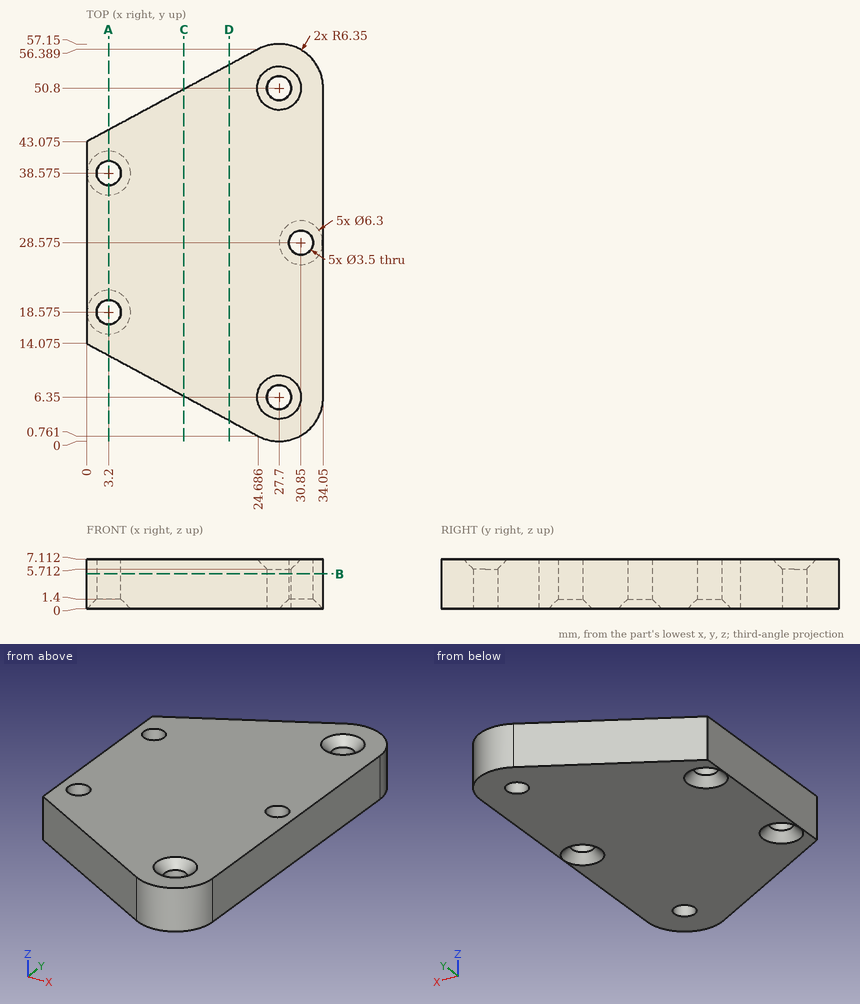
The drawing under review shows one solid part. Ordinate dimensions are in mm from its lowest x, y, z. Coordinates: 2 decimals unless noted, no trailing zeros. Order: outer loops, then holes, each group sorted by start corner. A loop starts at its lowest first (then second) coordinate and runs counter-clockwise, first axis right, second up. Notation, with made-up numbers: (61, 25.5) - (116, 25.5) arc R11 cw to (116, 39.5) - close; hole circle Ø2 at (61, 36). An arc over 180 degrees is marked (long way). Put each result on its own line as item: value.
1) Take a section at A-A, the plane x = 3.2. Give the boundary of the cut face in (y, z) (1 decimal).
Response values:
outline: (12.3, 0) - (15.4, 0) - (16.8, 1.4) - (16.8, 7.1) - (12.3, 7.1) - close; (20.3, 1.4) - (21.7, 0) - (35.4, 0) - (36.8, 1.4) - (36.8, 7.1) - (20.3, 7.1) - close; (40.3, 1.4) - (41.7, 0) - (44.8, 0) - (44.8, 7.1) - (40.3, 7.1) - close
2) Wall thickness on L1, parallel to Y at x = 27.7, z = 2.7; L2, parallel to X at y = 28.5, z = 1.25; L3, parallel to X at y = 5.5, z = 1.5 (1 decimal): over which ranges is each line inside the solid? List them lowest first. Write a range as from..to.
Response values:
L1: y = 0..4.6, 8.1..49.05, 52.55..57.15
L2: x = 0..28.95, 32.75..34.05
L3: x = 15.9..26.2, 29.2..34
3) Take a section at B-B, the plane z = 5. Count the separate pieces of the cut face and the enclosed holes in it, and give its area (3 significant figures).
Response values:
separate pieces: 1
enclosed holes: 5
area: 1,510 mm²
4) Take a section at D-D, the plane x = 20.5. Give the boundary of the cut face in (y, z).
Response values:
outline: (3.02, 0) - (54.13, 0) - (54.13, 7.11) - (3.02, 7.11) - close
5) Insertion check: P1, Ø4, axis at x = 8, z = 1.5, coming from the -Y side; P2, Ø1, axis at x = 25, z = 4, coming from the +Y side; P3, Ø3, axis at x = 20, z = 2.5, coming from the +Y side. Each pin has a flat end and moves straight along its axis. Give the tip position at first contact, or say it passes through.
Response values:
P1: stops at y = 8.68
P2: stops at y = 56.76
P3: stops at y = 54.67
6) Take a section at C-C, the plane x = 14. Give the boundary of the cut face in (y, z), and give its area (3 significant figures).
Response values:
outline: (6.52, 0) - (50.63, 0) - (50.63, 7.11) - (6.52, 7.11) - close
area: 314 mm²
